For this review, take the finished solid that the model builds, in its own axes (mm). Face numbers are marked on the shaded views. Round coordinates to 2 decimals unless told otherwise and drop trailing zeros. Write each loop counter-clockwise with the first axis right and the second up, starting at its lowest first coordinate (ties: lowest second). Pieces come first, ordered by that corner, then holes. Notation, with made-up numbers: (-37, -4) -> (8, -4) arc R26 ccw to (8, 23) -> close; hole circle Ø6 at (62, -14). An arc over 180 degrees is marked (long way). Answer in a Markdown table with one row per item.
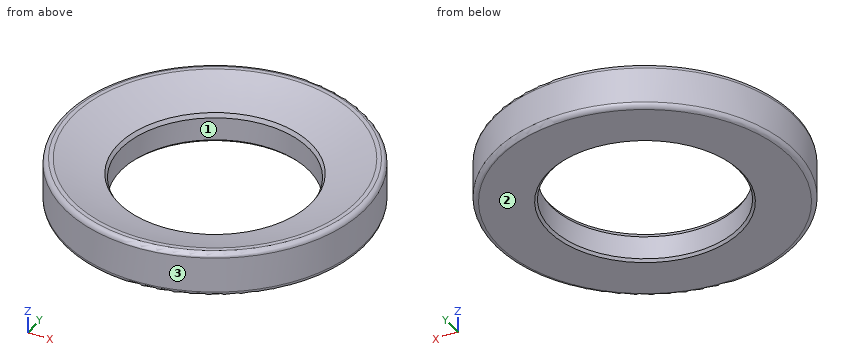
from build123d import *

# Parameters (mm, degrees)
FILLET2_R = 0.508


with BuildPart() as part:
    # Sketch1 → Revolve1 (revolve)
    with BuildSketch(Plane(origin=(0, 0, 0), x_dir=(0, 0, -1), z_dir=(1, 0, 0)), mode=Mode.PRIVATE) as revolve1_sk:
        with BuildLine():
            Line((39.8272, 15.875), (39.8272, 9.9314))
            Line((39.8272, 9.9314), (36.782839668, 9.9314))
            ThreePointArc((36.782839668, 9.9314), (36.004343784, 12.461830872), (35.052, 14.932089472))
            Line((35.052, 14.932089472), (35.052, 15.875))
            Line((35.052, 15.875), (39.8272, 15.875))
        make_face()
    revolve(revolve1_sk.sketch.rotate(Axis((0, 0, 0), (0, 0, -1)), 90), axis=Axis((0, 0, 0), (0, 0, -1)))

    # Chamfer1: read off the stored shape, not the designer's step
    # Chamfer1 outline → Chamfer1 (revolve, cut)
    with BuildSketch(Plane.XZ):
        Polygon((9.9314, -36.716530911), (9.9314, -37.142376439), (10.173807442, -36.716530911), align=None)
        Polygon((9.9314, -39.5732), (9.9314, -39.8272), (10.1854, -39.8272), align=None)
    revolve(axis=Axis((0, 0, 0), (0, 0, 1)), mode=Mode.SUBTRACT)

    # Fillet2
    fillet2_edges = [part.edges().sort_by_distance(p)[0] for p in [
        (-15.875, 0, -39.8272),
        (-15.875, 0, -35.052),
    ]]
    fillet(fillet2_edges, radius=FILLET2_R)


solid = part.part
1) Consider section B-B on z = -38.4. State the section outline as (x, y) points (3 decimals), then the cut area to 3 significant figures.
Solved:
| item | result |
|---|---|
| outline | circle Ø31.75 at (0, 0); hole circle Ø19.863 at (0, 0) |
| area | 482 mm² |
2) For line 1 (Y direction, x = 0, z = -37.9) (3 decimals); line 2 (X direction, y = 0.5, z = -39.1); line 3 (X direction, y = -3, z = -38.45), list the stretches that pass through material, from the lowest coordinate up. Write a range as [from, to].
Solved:
| item | result |
|---|---|
| line 1 | [-15.875, -9.931], [9.931, 15.875] |
| line 2 | [-15.87, -9.92], [9.92, 15.87] |
| line 3 | [-15.59, -9.47], [9.47, 15.59] |
3) Clearance check with flat-ended pins moving along their axes: pin 1 Ø8 at (x, y) = (-7, 6) entering from +Z; pin 2 Ø1 at (x, z) = (-12, -36) entering from -Y; pin 3 Ø2 at (x, z) = (6.5, -36) entering from +Y. State where each tip first meets the part, or that it passes through.
Solved:
| item | result |
|---|---|
| pin 1 | z = -35.73 |
| pin 2 | y = -10.94 |
| pin 3 | y = 14.89 |
4) Consider section A-A on x = 0. State the section outline as (y, z) points (3 decimals).
Solved:
| item | result |
|---|---|
| outline | (-15.875, -39.319) arc R0.508 ccw to (-15.367, -39.827) -> (-10.185, -39.827) -> (-9.931, -39.573) -> (-9.931, -37.142) -> (-10.174, -36.717) arc R38.1 cw to (-14.932, -35.052) -> (-15.367, -35.052) arc R0.508 ccw to (-15.875, -35.56) -> close; (9.931, -39.573) -> (10.185, -39.827) -> (15.367, -39.827) arc R0.508 ccw to (15.875, -39.319) -> (15.875, -35.56) arc R0.508 ccw to (15.367, -35.052) -> (14.932, -35.052) arc R38.1 cw to (10.174, -36.717) -> (9.931, -37.142) -> close |
5) Mouldability with a two-part tool opening along Y and no side actions: class the marked faces 1, 2 and 3 as pulls with the +Y half, pulls with the -Y half, needs draft (parallel to the pull), parting line crosses it, or undercut.
Solved:
| item | result |
|---|---|
| face 1 | undercut |
| face 2 | needs draft |
| face 3 | parting line crosses it |
